Autodesk Inventor part; units mm, degrees
ref_plane "YZ Plane" through (0, 0, 0) normal (1, 0, 0) x (0, 1, 0)
ref_plane "XZ Plane" through (0, 0, 0) normal (0, 1, 0) x (-1, 0, 0)
ref_plane "XY Plane" through (0, 0, 0) normal (0, 0, 1) x (1, 0, 0)
sketch "Sketch_1" plane through (0, 0, 0) normal (0, 0, 1) x (1, 0, 0)
  line L0 (5, 0) -> (0, 0)
  arc A0 (0, 7.65) -> (0.15, 7.5) centre (0.15, 7.65) ccw
  line L1 (0.15, 7.5) -> (4.85, 7.5)
  arc A1 (4.85, 7.5) -> (5, 7.65) centre (4.85, 7.65) ccw
  line L2 (5, 7.65) -> (5, 9.55)
  line L3 (5, 9.55) -> (0, 9.55)
  line L4 (0, 9.55) -> (0, 7.65)
revolve "Revolution1" add sketch "Sketch_1" angle 360 about axis through (5, 0, 0) along (1, 0, 0)
sketch "Sketch_2" plane through (0, 0, 0) normal (0, 0, 1) x (1, 0, 0)
  line L0 (3.5, 0) -> (1.5, 0)
  line L1 (1.0858, 9.8) -> (2.5, 8.3858)
  line L2 (2.5, 8.3858) -> (3.9142, 9.8)
  line L3 (3.9142, 9.8) -> (2.5, 11.2142)
  line L4 (2.5, 11.2142) -> (1.0858, 9.8)
revolve "Revolution2" cut sketch "Sketch_2" angle 360 about axis through (3.5, 0, 0) along (1, 0, 0)
properties part number "CRBT155A_PART1" material "ステンレス鋼"
Model file for the job. Use its own axes, mm. Coordinates: 2 decimals unless noted, no trailing zeros. Write each loop counter-clockwise with the first axis right and the second up, starting at its lowest first coordinate (ties: lowest second). Pieces come first, ordered by that corner, then holes. Notation, with made-up numbers: (-10.75, 69.5) - (34.25, 69.5) arc R21 cw to (34.25, 73.5) - close; hole circle Ø7 at (-10.5, 7). An arc over 180 degrees is marked (long way). Use a Markdown table: item, result. Add a question column.
Item 1: Drop a flat-ended pin along its axis: pin 1 (1.5 mm diameter, centred on x = 1, z = -2, fed in from -Y). Give the stop position or say it passes through.
Item 2: Band-saw the part on C-C, the plane x = 0.65. Write the cut outline in (y, z).
Item 3: Band-saw the part on A-A, the plane y = 0. Write the cut outline in (x, z), and give its area (3 significant figures).
Item 4: Drill centre lines: line 1 along Z through (x, y) = (1.2, 0); line 2 along Z through (x, y) = (2.85, 0); line 3 along Y through (x, z) = (1.05, 1.25). Where is each one in solid material? Low to high.
A:
| question | item | result |
|---|---|---|
| 1 | pin 1 | stops at y = -9.47 |
| 2 | outline | circle Ø19.1 at (0, 0); hole circle Ø15 at (0, 0) |
| 3 | outline | (0, -9.55) - (1.34, -9.55) - (2.5, -8.39) - (3.66, -9.55) - (5, -9.55) - (5, -7.65) arc R0.15 ccw to (4.85, -7.5) - (0.15, -7.5) arc R0.15 ccw to (0, -7.65) - close; (0, 7.65) arc R0.15 ccw to (0.15, 7.5) - (4.85, 7.5) arc R0.15 ccw to (5, 7.65) - (5, 9.55) - (3.66, 9.55) - (2.5, 8.39) - (1.34, 9.55) - (0, 9.55) - close |
| 3 | area | 17.8 mm² |
| 4 | line 1 | z = -9.55 to -7.5, 7.5 to 9.55 |
| 4 | line 2 | z = -8.74 to -7.5, 7.5 to 8.74 |
| 4 | line 3 | y = -9.47 to -7.4, 7.4 to 9.47 |
